```python
from build123d import *

# Parameters (mm, degrees)
SKICA1_W                 = 54.6
SKICA1_H                 = 54.6
SKICA1_R                 = 2.3
P_IDAT_VYSUNUT_M1_DEPTH  = 1.7
SKICA2_W                 = 54.6
SKICA2_H                 = 54.6
P_IDAT_VYSUNUT_M2_DEPTH  = 1
SKICA3_R                 = 2.3
P_IDAT_VYSUNUT_M3_DEPTH  = 1.6
SKICA4_W                 = 13.54
SKICA4_H                 = 26.5
SKICA4_W_2               = 19
SKICA4_H_2               = 44
SKICA4_W_3               = 18.04
SKICA4_H_3               = 37.5
P_IDAT_VYSUNUT_M4_DEPTH  = 4
SKICA5_W                 = 8
SKICA5_H                 = 4
ODEBRAT_VYSUNUT_M1_DEPTH = 6
SKICA6_W                 = 8
SKICA6_H                 = 4
ODEBRAT_VYSUNUT_M2_DEPTH = 6
SKICA7_W                 = 2
SKICA7_H                 = 8
ODEBRAT_VYSUNUT_M3_DEPTH = 38
SKICA8_W                 = 2
SKICA8_H                 = 8
ODEBRAT_VYSUNUT_M4_DEPTH = 13
SKICA11_W                = 16.5
SKICA11_H                = 36.5
SKICA11_W_2              = 18
SKICA11_H_2              = 43
SKICA11_W_3              = 12
SKICA11_H_3              = 25.5
ODEBRAT_VYSUNUT_M5_DEPTH = 4


with BuildPart() as part:
    # Skica1 → Přidat vysunutím1 (new body)
    with BuildSketch(Plane.XY):
        Rectangle(SKICA1_W, SKICA1_H)
        with Locations((-23.4, 23.4)):
            Circle(SKICA1_R, mode=Mode.SUBTRACT)
        with Locations((23.4, 23.4)):
            Circle(SKICA1_R, mode=Mode.SUBTRACT)
        with Locations((-23.4, -23.4)):
            Circle(SKICA1_R, mode=Mode.SUBTRACT)
        with Locations((23.4, -23.4)):
            Circle(SKICA1_R, mode=Mode.SUBTRACT)
    extrude(amount=P_IDAT_VYSUNUT_M1_DEPTH)

    # Skica2 → Přidat vysunutím2 (add)
    with BuildSketch(Plane.XY.offset(1.7)):
        Rectangle(SKICA2_W, SKICA2_H)
    extrude(amount=P_IDAT_VYSUNUT_M2_DEPTH)

    # Skica3 → Přidat vysunutím3 (add)
    with BuildSketch(Plane.XY.offset(2.7)):
        with Locations((-23.4, 23.4)):
            Circle(SKICA3_R)
        with Locations((23.4, 23.4)):
            Circle(SKICA3_R)
        with Locations((-23.4, -23.4)):
            Circle(SKICA3_R)
        with Locations((23.4, -23.4)):
            Circle(SKICA3_R)
    extrude(amount=P_IDAT_VYSUNUT_M3_DEPTH)

    # Skica4 → Přidat vysunutím4 (add)
    with BuildSketch(Plane.XY.offset(2.7)):
        with Locations((18.53, 1.14272147)):
            Rectangle(SKICA4_W, SKICA4_H)
        with Locations((2.25, -0.25)):
            Rectangle(SKICA4_W_2, SKICA4_H_2)
        with Locations((-16.28, 0.55)):
            Rectangle(SKICA4_W_3, SKICA4_H_3)
    extrude(amount=P_IDAT_VYSUNUT_M4_DEPTH)

    # Skica5 → Odebrat vysunutím1 (cut)
    with BuildSketch(Plane(origin=(0, -22.25, 0), x_dir=(-1, 0, 0), z_dir=(0, -1, 0))):
        with Locations((-2, -4.7)):
            Rectangle(SKICA5_W, SKICA5_H)
    extrude(amount=-ODEBRAT_VYSUNUT_M1_DEPTH, mode=Mode.SUBTRACT)

    # Skica6 → Odebrat vysunutím2 (cut)
    with BuildSketch(Plane(origin=(0, 21.75, 0), x_dir=(1, 0, 0), z_dir=(0, 1, 0))):
        with Locations((2, -4.7)):
            Rectangle(SKICA6_W, SKICA6_H)
    extrude(amount=-ODEBRAT_VYSUNUT_M2_DEPTH, mode=Mode.SUBTRACT)

    # Skica7 → Odebrat vysunutím3 (cut)
    with BuildSketch(Plane.ZY.offset(25.3)):
        with Locations((3.7, -12.2)):
            Rectangle(SKICA7_W, SKICA7_H)
        with Locations((3.7, 9.3)):
            Rectangle(SKICA7_W, SKICA7_H)
    extrude(amount=-ODEBRAT_VYSUNUT_M3_DEPTH, mode=Mode.SUBTRACT)

    # Skica8 → Odebrat vysunutím4 (cut)
    with BuildSketch(Plane(origin=(25.3, 0, 0), x_dir=(0, 0, -1), z_dir=(1, 0, 0))):
        with Locations((-3.7, 0.89272147)):
            Rectangle(SKICA8_W, SKICA8_H)
    extrude(amount=-ODEBRAT_VYSUNUT_M4_DEPTH, mode=Mode.SUBTRACT)

    # Skica11 → Odebrat vysunutím5 (cut)
    with BuildSketch(Plane.XY.offset(6.7)):
        with Locations((-16.55, 0.55)):
            Rectangle(SKICA11_W, SKICA11_H)
        with Locations((2.25, -0.25)):
            Rectangle(SKICA11_W_2, SKICA11_H_2)
        with Locations((18.26, 1.14272147)):
            Rectangle(SKICA11_W_3, SKICA11_H_3)
    extrude(amount=-ODEBRAT_VYSUNUT_M5_DEPTH, mode=Mode.SUBTRACT)


solid = part.part
```
The model under review builds one solid part; all positions refer to its coordinate system, in mm. A direction names the side the tool comes from. Round coordinates to 2 decimals unless told otherwise and drop trailing zeros. Loops run counter-clockwise (first coordinate to the right, second up) from the corner with the lowest first, then second, coordinate; pieces in that order, holes last. Notation, with made-up numbers: M -1,55.25 L 48,55.25 A12 cw 48,76.25 Z; hole C 75.25,89 d11. An arc over 180 degrees is marked long. Answer as a JSON object with one key per item and string values.
(1) Draft analysis for pull direction X (two halves, no side actions). For faces 1 (the flat face through (-8, 1, 6.7)), 2 (the flat face through (9, -22.25, 5)), state which applies: released by +X, released by -X, zero draft, split by the parting line, or undercut.
Resolved:
{"face 1": "zero draft", "face 2": "undercut"}
(2) Take a section at C-C on z = 1. Give the boundary of the cut face in (x, y).
Resolved:
{"outline": "M -27.3,-27.3 L 27.3,-27.3 L 27.3,27.3 L -27.3,27.3 Z; hole C -23.4,-23.4 d4.6; hole C -23.4,23.4 d4.6; hole C 23.4,-23.4 d4.6; hole C 23.4,23.4 d4.6"}
(3) Clearance check with flat-ended pins moving along their axes: P1, Ø1.1, axis at x = -7.5, z = 4, coming from the -Y side; P2, Ø1.1, axis at x = -8, z = 4, coming from the +Y side; P3, Ø1.5, axis at y = 1, z = 3.5, coming from the +X side. State where each tip first meets the part, or that it passes through.
Resolved:
{"P1": "y = -22.25", "P2": "y = 19.3", "P3": "x = 12.26"}
(4) Take a section at A-A on y = -13. Give the boundary of the cut face in (x, z).
Resolved:
{"outline": "M -27.3,0 L 27.3,0 L 27.3,2.7 L -27.3,2.7 Z; M -25.3,4.7 L -24.8,4.7 L -24.8,6.7 L -25.3,6.7 Z; M -8.3,4.7 L -7.26,4.7 L -7.26,6.7 L -8.3,6.7 Z; M -7.25,4.7 L -6.75,4.7 L -6.75,6.7 L -7.25,6.7 Z; M 11.25,4.7 L 11.75,4.7 L 11.75,6.7 L 11.25,6.7 Z"}
(5) Tool access review of faces 3 (the flat face through (18, -12.107, 5)), 4 (the flat face through (23, -23, 4.3)), 5 (the cylindrical face through (21.102, 23.501, 0.838)), 6 (the flat face through (-17, 18.8, 5)): name each direction out of +Z, -Z, +X, -X, +Y, -Y from which nothing blocks a thin tool from reaching the whole face with its end or side.
Resolved:
{"face 3": "+Z, +X", "face 4": "+Z, +X, -Y", "face 5": "-Z", "face 6": "+Z"}
(6) To check wall thickness, follow line 1 along Y through (x, z) = (23.4, 0.6); line 2 along Y through (x, z) = (11.5, 4.25); line 3 along Y through (x, z) = (-23, 5.75). State the ranges of each line that lie inside material, in increasing order.
Resolved:
{"line 1": "-27.3 to -25.7, -21.1 to 21.1, 25.7 to 27.3", "line 2": "-22.25 to -16.2, -8.2 to 5.3, 13.3 to 21.75", "line 3": "-18.2 to -17.7, 18.8 to 19.3"}
(7) Take a section at D-D on x = 9. Give the boundary of the cut face in (y, z), and give its area (3 significant figures).
Resolved:
{"outline": "M -27.3,0 L 27.3,0 L 27.3,2.7 L 21.75,2.7 L 21.75,6.7 L 21.25,6.7 L 21.25,2.7 L -21.75,2.7 L -21.75,6.7 L -22.25,6.7 L -22.25,2.7 L -27.3,2.7 Z", "area": "151 mm²"}
(8) Take a section at B-B on z = 5.5. Count the separate pieces of the cut face and the enclosed holes in it, and give its area (3 significant figures).
Resolved:
{"separate pieces": "4", "enclosed holes": "2", "area": "181 mm²"}
